from build123d import *

# Parameters (mm, degrees)
F2_R     = 2.032
F3_DEPTH = 15.875
F4_DEPTH = 10.2362


# Not quite as in the source:
# - a feature names something its author has since deleted; it is built from what else it names


with BuildPart() as f1:
    # F0 (on Top) → F1 (revolve)
    with BuildSketch(Plane.XY):
        with BuildLine():
            Line((0, -5.1666409709), (0, -12.1516409709))
            Line((0, -12.1516409709), (45.72, -12.1516409709))
            ThreePointArc((45.72, -12.1516409709), (42.9147529825, -8.6591409709), (45.72, -5.1666409709))
            Line((45.72, -5.1666409709), (0, -5.1666409709))
        make_face()
    revolve(axis=Axis((0, -8.561744864, 0), (0, 1, 0)))

    # F2 (on Front) → F3 (cut)
    with BuildSketch(Plane.XZ):
        with BuildLine():
            Line((13.97, 3.6661742094), (13.97, -3.6661742094))
            Line((13.97, -3.6661742094), (38.6802071591, -16.0932599922))
            ThreePointArc((38.6802071591, -16.0932599922), (41.8782799617, 1.5705660984), (37.3345500424, 18.9369975174))
            Line((37.3345500424, 18.9369975174), (13.97, 3.6661742094))
        make_face()
        with BuildLine():
            Line((3.81, 41.7094333604), (3.81, 13.9314619955))
            Line((3.81, 13.9314619955), (10.16, 10.2652877862))
            Line((10.16, 10.2652877862), (34.2119266748, 24.1516741264))
            ThreePointArc((34.2119266748, 24.1516741264), (20.9542761873, 36.2954737188), (3.81, 41.7094333604))
        make_face()
        with BuildLine():
            Line((-34.2388233597, 24.0958361272), (-10.16, 10.2652877862))
            Line((-10.16, 10.2652877862), (-3.81, 13.9314619955))
            Line((-3.81, 13.9314619955), (-3.81, 41.7173788368))
            ThreePointArc((-3.81, 41.7173788368), (-20.9781685322, 36.2803485402), (-34.2388233597, 24.0958361272))
        make_face()
        with BuildLine():
            Line((-38.6893950171, -16.0623838358), (-13.97, -3.6661742094))
            Line((-13.97, -3.6661742094), (-13.97, 3.6661742094))
            Line((-13.97, 3.6661742094), (-37.3405062231, 18.9372899969))
            ThreePointArc((-37.3405062231, 18.9372899969), (-41.8787701809, 1.5863648371), (-38.6893950171, -16.0623838358))
        make_face()
        with BuildLine():
            Line((-3.81, -13.9314619955), (-10.16, -10.2652877862))
            Line((-10.16, -10.2652877862), (-34.3038742814, -23.844345572))
            ThreePointArc((-34.3038742814, -23.844345572), (-20.4303998238, -36.5921428083), (-2.2874128339, -41.6726596109))
            Line((-2.2874128339, -41.6726596109), (-3.81, -13.9314619955))
        make_face()
        with BuildLine():
            Line((10.16, -10.2652877862), (3.81, -13.9314619955))
            Line((3.81, -13.9314619955), (5.4400267393, -41.5192010913))
            ThreePointArc((5.4400267393, -41.5192010913), (22.3730839146, -35.4381883413), (35.1536490306, -22.7746857971))
            Line((35.1536490306, -22.7746857971), (10.16, -10.2652877862))
        make_face()
        Circle(F2_R)
    extrude(amount=F3_DEPTH, mode=Mode.SUBTRACT)

    # F2 (on Front) → F4 (cut)
    with BuildSketch(Plane.XZ):
        Polygon((-7.0386894402, 0.071686571), (-3.5814271117, -6.059840579), (3.4572623285, -6.1315271501), (7.0386894402, -0.071686571), (3.5814271117, 6.059840579), (-3.4572623285, 6.1315271501), align=None)
        Circle(F2_R, mode=Mode.SUBTRACT)
    extrude(amount=F4_DEPTH, mode=Mode.SUBTRACT)


solid = f1.part
Verification items for the finished model (mm, model axes). A direction names the side the tool comes from. Round coordinates to 2 decimals unless told otherwise and drop trailing zeros. Order: outer loops, then holes, each group sorted by start corner. A loop starts at its lowest first (then second) coordinate and runs counter-clockwise, first axis right, second up.
1. Release check for a two-part mould opening along X. For faces 3 (the cylindrical face through (-20.663, -8.61, -36.462)), 4 (the cylindrical face through (-41.87, -8.61, 1.84)) record: +X half, -X half, draft (parallel to the pull), parting line (faces both ways), or undercut.
Final values:
face 3: undercut
face 4: undercut
2. Access from +Z, -Z, +X, -X, +Y, -Y to the whole of each face (thin tool, end or side, straight path). Record for faces 1 (the flat face through (22, -8.6, 17.1)), 2 (the flat face through (5.334, -7.666, 2.951)).
Final values:
face 1: +Y, -Y
face 2: +Y
3. Section check B-B on x = 0. Record the cut outline in (y, z), then the cut area to 3 significant figures.
Final values:
outline: (-12.15, -45.72) arc R3.58 cw to (-5.17, -45.72) - (-5.17, -6.1) - (-10.24, -6.1) - (-10.24, -2.03) - (-12.15, -2.03) - close; (-12.15, 2.03) - (-10.24, 2.03) - (-10.24, 6.1) - (-5.17, 6.1) - (-5.17, 45.72) arc R3.58 cw to (-12.15, 45.72) - close
area: 540 mm2
4. Thickness scan on L1, parallel to X at y = -11.1, z = 0; L2, parallel to Z at x = -6.5, y = -6; L3, parallel to X at y = -10.8, z = 0. Record the ranges inside material, lowest first.
Final values:
L1: x = -43.88 to -41.91, -13.97 to -2.03, 2.03 to 13.97, 41.91 to 43.88
L2: z = -43.62 to -41.29, -12.38 to -0.88, 0.98 to 12.38, 41.39 to 43.62
L3: x = -43.63 to -41.91, -13.97 to -2.03, 2.03 to 13.97, 41.91 to 43.63
5. Go/stop test with flat-tipped pins: P1, Ø2, axis at y = -8, z = -1, coming from the -X side; P2, Ø1.5, axis at x = 35.5, y = -8, coming from the -Z side; P3, Ø1.5, axis at y = -7, z = 3.5, coming from the -X side. Record where each tip stops, or that it passes through.
Final values:
P1: stops at x = -43.31
P2: stops at z = -25.32
P3: stops at x = -43.71
6. Section check A-A on y = -8.75. State how many separate pieces and enclosed holes the cut face has, then the cut area to 3 significant figures.
Final values:
separate pieces: 1
enclosed holes: 7
area: 2,020 mm2
